```python
from build123d import *


with BuildPart() as part:
    # Sketch1 → Revolve1 (revolve)
    with BuildSketch(Plane.XY, mode=Mode.PRIVATE) as revolve1_sk:
        Polygon((12.7, -12.6873), (33.528, -13.335), (33.528, -16.764), (12.7, -16.764), align=None)
    revolve(revolve1_sk.sketch.rotate(Axis((-22.402366391, 0, 0), (1, 0, 0)), 270), axis=Axis((-22.402366391, 0, 0), (1, 0, 0)))

    # Sketch2 → Revolve2 (revolve)
    with BuildSketch(Plane.XY, mode=Mode.PRIVATE) as revolve2_sk:
        Polygon((-16.764, 33.528), (-16.764, 12.7), (-12.6873, 12.7), (-13.335, 33.528), align=None)
    revolve(revolve2_sk.sketch.rotate(Axis((0, 0, 0), (0, 1, 0)), 270), axis=Axis((0, 0, 0), (0, 1, 0)))


solid = part.part
```
Source: CAD feature listing. Evaluate the final solid. Frame: model axes, mm. A direction names the side the tool comes from. Give positions to 0.01 mm unless a question says otherwise; leave off trailing zeros. Write each loop counter-clockwise with the first axis right and the second up, starting at its lowest first coordinate (ties: lowest second). Pieces come first, ordered by that corner, then holes.
1. Section query C-C (z = 0). Return the cut outline in (x, y) (3 decimals), then the cut area to 3 significant figures.
2. Section query A-A (z = -14). Return the cut outline in (x, y), then the cut area to 3 significant figures.
3. First-contact query: pin 1 (3 mm diameter, centred on y = 24, z = 8.5, fed in from -X); pin 2 (3.5 mm diameter, centred on x = 14, z = -0.5, fed in from -Y); pin 3 (1.5 mm diameter, centred on x = 28.5, z = -9, fed in from -Y); pin 4 (3 mm diameter, centred on x = 16, y = 28, fed in from +Z). Flat tips, straight axial feed; report the tip coordinate or a pass-through.
4. Material intervals for line 1 along Y through (x, z) = (28.5, 1.5); line 2 along X through (y, z) = (10, 12.5); line 3 along X through (y, z) = (21.5, 10), sorted ascending.
5. Pull-direction query (Z, two-part tool) for faces 5 (the face through (12.7, -13, 1)), 6 (the face through (-3.91, 23.11, -12.41)), 7 (the face through (-16.62, 22.97, 2.18)), 8 (the face through (15, 12.7, 0)); classes: +Z half, -Z half, draft (parallel to the pull), parting line (faces both ways), or undercut.
6. Access query for faces 1 (the face through (22.97, -16.62, -2.18)), 2 (the face through (-13, 12.7, -1)), 3 (the face through (33.528, 7.4, 11.3)), 4 (the face through (12.7, 15, 0)). Directions: +Z, -Z, +X, -X, +Y, -Y. A direction counts if a zero-diameter tool reaches every point of the face in a straight line with its end or side. Return the directions, or none.
7. Section query D-D (y = 16). Return the cut outline in (x, z), then the cut area to 3 significant figures.
8. Section query B-B (x = 0). Return the cut outline in (y, z) (3 decimals), then the cut area to 3 significant figures.
Output values:
1. outline: (-16.764, 12.7) - (-12.687, 12.7) - (-13.335, 33.528) - (-16.764, 33.528) - close; (12.687, 12.7) - (12.7, 12.7) - (12.7, 12.687) - (13.108, 12.7) - (16.764, 12.7) - (16.764, 12.814) - (33.528, 13.335) - (33.528, 16.764) - (16.764, 16.764) - (16.764, 33.528) - (13.335, 33.528) - (12.814, 16.764) - (12.7, 16.764) - (12.7, 13.108) - close; (12.7, -16.764) - (33.528, -16.764) - (33.528, -13.335) - (12.7, -12.687) - close
1. area: 297 mm2
2. outline: (-9.22, 12.7) - (9.22, 12.7) - (9.22, 33.53) - (-9.22, 33.53) - close; (12.7, -9.22) - (33.53, -9.22) - (33.53, 9.22) - (12.7, 9.22) - close
2. area: 768 mm2
3. pin 1: stops at x = -15.23
3. pin 2: stops at y = -16.76
3. pin 3: stops at y = -14.59
3. pin 4: stops at z = 8.41
4. line 1: y = -16.7 to -13.09, 13.09 to 16.7
4. line 2: x = 12.7 to 33.53
4. line 3: x = -13.45 to -8.25, 8.25 to 13.45
5. face 5: draft
5. face 6: undercut
5. face 7: parting line
5. face 8: undercut
6. face 1: +X
6. face 2: +Z, -Z, -X, -Y
6. face 3: +Z, -Z, +X, +Y, -Y
6. face 4: +Y
7. outline: (16, -5) - (33.53, -5) - (33.53, 5) - (16, 5) arc R16.76 ccw (long way) to start; hole (12.7, -1.51) - (12.7, 1.51) arc R12.79 ccw (long way) to start
7. area: 539 mm2
8. outline: (12.7, -16.764) - (33.528, -16.764) - (33.528, -13.335) - (12.7, -12.687) - close; (12.7, 12.687) - (33.528, 13.335) - (33.528, 16.764) - (12.7, 16.764) - close
8. area: 156 mm2
